Design review of the part built by this model. Coordinates are the model's own, in mm. A direction names the side the tool comes from. Coordinates: 2 decimals unless noted, no trailing zeros. Write each loop counter-clockwise with the first axis right and the second up, starting at its lowest first coordinate (ties: lowest second). Pieces come first, ordered by that corner, then holes.
Q1. Machinability: for faces 1 (the flat face through (4.03, 7.4, -2.76)), 2 (the flat face through (0.86, 7.4, -4.85)), 3 (the flat face through (-3.09, 7.4, 3.79)), 4 (the flat face through (-4.93, 7.4, -0.16)), which of the approach directions +Z, -Z, +X, -X, +Y, -Y give a long, thin tool a straight path to every point of the face, cutting with its end or side? Answer none if there is none.
Q2. For probe 1 along Z at (x, y) = (0, 3.5); probe 2 along X at (y, z) = (5.25, -3.25); probe 3 along Z at (x, y) = (-5.5, 9), list the stretches that pass through material, from the lowest coordinate up.
Q3. Insertion check: pin 1 (2 mm diameter, centred on y = 7.5, z = -1.5, fed in from -X); pin 2 (1.3 mm diameter, centred on x = 0, y = 10.5, fed in from -Z); pin 3 (1 mm diameter, centred on y = 4, z = -4, fed in from +X). Each pin has a flat end and moves straight along its axis. Give the tip position at first contact, or say it passes through.
Q4. Take a section at B-B (x = -4.25). Give the boundary of the cut face in (y, z).
Q5. Mouldability with a two-part tool opening along X and no side actions: class faces 5 (the flat face through (-4.06, 7.4, -2.8)), 6 (the flat face through (4.68, 7.4, 1.54)), 7 (the flat face through (3.35, 7.4, -3.62)), 8 (the flat face through (0.542, 7.395, 4.899)) as pulls with the +X half, pulls with the -X half, needs draft (parallel to the pull), parting line crosses it, or undercut.
Q6. Take a section at A-A (z = 0). Give the boundary of the cut face in (x, y).
```python
from build123d import *

# Parameters (mm, degrees)
ESBO_O1_W                = 1.9
ESBO_O1_H                = 15
RESSALTO_EXTRUS_O1_DEPTH = 15
PADR_OCIRCULAR1_COUNT    = 11
RESSALTO_EXTRUS_O2_DEPTH = 15


with BuildPart() as part:
    # Esboço1 → Revolução1 (revolve)
    with BuildSketch(Plane.XY):
        with Locations((2.55, 7.5)):
            Rectangle(ESBO_O1_W, ESBO_O1_H)
    revolve(axis=Axis((0, 0, 0), (0, 1, 0)))

    # Esboço3 → Ressalto-extrusão1 (add)
    with BuildSketch(Plane(origin=(0, 0, 0), x_dir=(-1, 0, 0), z_dir=(0, -1, 0))):
        with BuildLine():
            Line((-0.194663871, -6.374258983), (-0.9, -3.382306905))
            ThreePointArc((-0.9, -3.382306905), (0, -3.5), (0.9, -3.382306905))
            Line((0.9, -3.382306905), (0.194663871, -6.374258983))
            ThreePointArc((0.194663871, -6.374258983), (0, -6.528368053), (-0.194663871, -6.374258983))
        make_face()
    extrude(amount=-RESSALTO_EXTRUS_O1_DEPTH)

    # PadrãoCircular1: part ×11 about axis
    padr_ocircular1_axis = Axis((0, 0, 0), (0, 1, 0))


with BuildPart() as part_1:
    add(part.part)
    for i in range(1, PADR_OCIRCULAR1_COUNT):
        add(part.part.rotate(padr_ocircular1_axis, i * 360 / PADR_OCIRCULAR1_COUNT))

    # Esboço4 → Ressalto-extrusão2 (add)
    with BuildSketch(Plane.XZ):
        with BuildLine():
            Line((1.322875656, 0.9), (-1.322875656, 0.9))
            ThreePointArc((-1.322875656, 0.9), (0, 1.6), (1.322875656, 0.9))
        make_face()
    extrude(amount=-RESSALTO_EXTRUS_O2_DEPTH)


solid = part_1.part
```
Response:
1. face 1: +X, +Y, -Y
1. face 2: -Z, +Y, -Y
1. face 3: +Y, -Y
1. face 4: -X, +Y, -Y
2. probe 1: z = -3.5 to -1.6, 0.9 to 6.53
2. probe 2: x = -4.38 to -2.64, -1.83 to 1.83, 2.64 to 4.38
2. probe 3: z = -1.17 to -0.39, 2.18 to 2.78
3. pin 1: stops at x = -6.46
3. pin 2: stops at z = -4.48
3. pin 3: stops at x = 4.98
4. outline: (0, -4.09) - (15, -4.09) - (15, -3.06) - (0, -3.06) - close; (0, -1.28) - (15, -1.28) - (15, 0.11) - (0, 0.11) - close; (0, 1.21) - (15, 1.21) - (15, 2.53) - (0, 2.53) - close
5. face 5: pulls with the -X half
5. face 6: pulls with the +X half
5. face 7: undercut
5. face 8: undercut
6. outline: (-4.52, 0) - (-1.6, 0) - (-1.6, 15) - (-4.52, 15) - close; (1.6, 0) - (4.52, 0) - (4.52, 15) - (1.6, 15) - close
